```python
from build123d import *

# Parameters (mm, degrees)
SKETCH1_R           = 15
BOSS_EXTRUDE1_DEPTH = 7
SKETCH2_R           = 17.5
BOSS_EXTRUDE2_DEPTH = 3
SKETCH3_R           = 1.5
CUT_EXTRUDE1_DEPTH  = 10
SKETCH5_R           = 2.5
CUT_EXTRUDE3_DEPTH  = 3
CUT_EXTRUDE5_DEPTH  = 10


with BuildPart() as part:
    # Sketch1 → Boss-Extrude1 (new body)
    with BuildSketch(Plane.XY):
        Circle(SKETCH1_R)
    extrude(amount=BOSS_EXTRUDE1_DEPTH)

    # Sketch2 → Boss-Extrude2 (add)
    with BuildSketch(Plane.XY.offset(7)):
        Circle(SKETCH2_R)
    extrude(amount=BOSS_EXTRUDE2_DEPTH)

    # Sketch3 → Cut-Extrude1 (cut)
    with BuildSketch(Plane.XY.offset(10)):
        with Locations((-11, 0)):
            Circle(SKETCH3_R)
        with Locations((11, 0)):
            Circle(SKETCH3_R)
    extrude(amount=-CUT_EXTRUDE1_DEPTH, mode=Mode.SUBTRACT)

    # Sketch5 → Cut-Extrude3 (cut)
    with BuildSketch(Plane.XY.offset(10)):
        with Locations((11, 0)):
            Circle(SKETCH5_R)
        with Locations((-11, 0)):
            Circle(SKETCH5_R)
    extrude(amount=-CUT_EXTRUDE3_DEPTH, mode=Mode.SUBTRACT)

    # Sketch4 → Cut-Extrude5 (cut)
    with BuildSketch(Plane.XY.offset(10)):
        with BuildLine():
            Line((-1.389019438, 1.575), (1.389019438, 1.575))
            ThreePointArc((1.389019438, 1.575), (0, -2.1), (-1.389019438, 1.575))
        make_face()
    extrude(amount=-CUT_EXTRUDE5_DEPTH, mode=Mode.SUBTRACT)


solid = part.part
```
Verification items for the finished model (mm, model axes). A direction names the side the tool comes from. Round coordinates to 2 decimals unless told otherwise and drop trailing zeros. Write each loop counter-clockwise with the first axis right and the second up, starting at its lowest first coordinate (ties: lowest second). Pieces come first, ordered by that corner, then holes. Notation, with made-up numbers: (13, 31.5) -> (70, 31.5) arc R3 ccw to (70, 35.5) -> close; hole circle Ø9 at (-31.5, -4.5). An arc over 180 degrees is marked (long way). Write each question's results on one line, items separated by ' | '.
Q1. Sectioned sample at C-C, the plane z = 2.25. Record the boundary of the cut face in (x, y) (3 decimals), and give its area (3 significant figures).
Derived:
outline: circle Ø30 at (0, 0); hole circle Ø3 at (-11, 0); hole (-1.389, 1.575) arc R2.1 ccw (long way) to (1.389, 1.575) -> close; hole circle Ø3 at (11, 0) | area: 680 mm²
Q2. Sectioned sample at A-A, the plane x = 0. Record the boundary of the cut face in (y, z) (3 decimals), and give its area (3 significant figures).
Derived:
outline: (-17.5, 7) -> (-15, 7) -> (-15, 0) -> (-2.1, 0) -> (-2.1, 10) -> (-17.5, 10) -> close; (1.575, 0) -> (15, 0) -> (15, 7) -> (17.5, 7) -> (17.5, 10) -> (1.575, 10) -> close | area: 278 mm²
Q3. Access from +Z, -Z, +X, -X, +Y, -Y to the whole of each face (thin tool, end or side, straight path). Record for faces 4 (the face through (-13.5, 0.1, 8.5)), 5 (the face through (13, 8, 7)), 6 (the face through (-13.887, -10.648, 8.479)).
Derived:
face 4: +Z | face 5: -Z | face 6: +Z, -Z
Q4. Sectioned sample at B-B, the plane y = 0. Record the boundary of the cut face in (x, z), and give its area (3 significant figures).
Derived:
outline: (-17.5, 7) -> (-15, 7) -> (-15, 0) -> (-12.5, 0) -> (-12.5, 7) -> (-13.5, 7) -> (-13.5, 10) -> (-17.5, 10) -> close; (-9.5, 0) -> (-2.1, 0) -> (-2.1, 10) -> (-8.5, 10) -> (-8.5, 7) -> (-9.5, 7) -> close; (2.1, 0) -> (9.5, 0) -> (9.5, 7) -> (8.5, 7) -> (8.5, 10) -> (2.1, 10) -> close; (12.5, 0) -> (15, 0) -> (15, 7) -> (17.5, 7) -> (17.5, 10) -> (13.5, 10) -> (13.5, 7) -> (12.5, 7) -> close | area: 201 mm²
Q5. Go/stop test with flat-tipped pins: pin 1 Ø2 at (x, z) = (0.5, 5) entering from -Y; pin 2 Ø4 at (y, z) = (-11.5, 1) entering from +X; pin 3 Ø3 at (x, z) = (-12.5, 7.5) entering from -Y. Record where each tip stops, or that it passes through.
Derived:
pin 1: stops at y = -15 | pin 2: stops at x = 11.61 | pin 3: stops at y = -13.61
Q6. Thickness scan on probe 1 along Y at (x, z) = (0, 3.25) (3 decimals); probe 2 along X at (y, z) = (-9, 7.75); probe 3 along X at (y, z) = (1, 5.25). Record the ranges inside material, lowest first.
Derived:
probe 1: y = -15 to -2.1, 1.575 to 15 | probe 2: x = -15.01 to 15.01 | probe 3: x = -14.97 to -12.12, -9.88 to -1.85, 1.85 to 9.88, 12.12 to 14.97
Q7. Draft check along Y on faces 1 (the face through (0, 1.575, 5)), 2 (the face through (-14.985, 0.66, 3.451)), 3 (the face through (0, -4, 10)). Enter one of: released by +Y, released by -Y, zero draft, split by the parting line, or undercut.
Derived:
face 1: undercut | face 2: split by the parting line | face 3: zero draft
Q8. Sectioned sample at D-D, the plane y = 13.5. Record the boundary of the cut face in (x, z), and give its area (3 significant figures).
Derived:
outline: (-11.14, 7) -> (-6.54, 7) -> (-6.54, 0) -> (6.54, 0) -> (6.54, 7) -> (11.14, 7) -> (11.14, 10) -> (-11.14, 10) -> close | area: 158 mm²
